from build123d import *

# Parameters (mm, degrees)
F0_R     = 4.953
F1_DEPTH = 4.7752
F2_DEPTH = 6.35
F4_DEPTH = 1.5748
F5_SIZE2 = 1.57479
F5_SIZE  = 3.17499
F6_SIZE  = 1.57479
F7_R     = 9.525
F8_R     = 4.953
F9_DEPTH = 6.35
F11_D    = 9.92124


# Not quite as in the source:
# - a fillet or chamfer is up to 0.001 mm smaller than in the source, because OpenCascade refuses the exact size


with BuildPart() as f1:
    # F0 (on Front) → F1 (new body)
    with BuildSketch(Plane.XZ):
        Polygon((0, 31.75), (0, 0), (25.4, 0), (25.4, 31.75), (12.7, 31.75), align=None)
        with BuildLine():
            ThreePointArc((22.225, 22.225), (5.9648079092, 15.4898079092), (12.7, 31.75))
            ThreePointArc((12.7, 31.75), (19.4351920908, 28.9601920908), (22.225, 22.225))
        make_face(mode=Mode.SUBTRACT)
        with BuildLine():
            ThreePointArc((22.225, 22.225), (19.4351920908, 28.9601920908), (12.7, 31.75))
            ThreePointArc((12.7, 31.75), (5.9648079092, 15.4898079092), (22.225, 22.225))
        make_face()
        with Locations((12.7, 22.225)):
            Circle(F0_R, mode=Mode.SUBTRACT)
    extrude(amount=F1_DEPTH)

    # F0 (on Front) → F2 (join)
    with BuildSketch(Plane.XZ):
        with BuildLine():
            ThreePointArc((22.225, 22.225), (19.4351920908, 28.9601920908), (12.7, 31.75))
            ThreePointArc((12.7, 31.75), (5.9648079092, 15.4898079092), (22.225, 22.225))
        make_face()
        with Locations((12.7, 22.225)):
            Circle(F0_R, mode=Mode.SUBTRACT)
    extrude(amount=F2_DEPTH)

    # F3 (on face) → F4 (join, through all)
    with BuildSketch(Plane.XZ.offset(6.35)):
        with BuildLine():
            ThreePointArc((25.4, 10.2581491177), (12.7, 4.7752), (0, 10.2581491177))
            Line((0, 10.2581491177), (0, 0))
            Line((0, 0), (25.4, 0))
            Line((25.4, 0), (25.4, 10.2581491177))
        make_face()
    extrude(amount=-F4_DEPTH)

    # F5 (size 3.175 and 1.5748 in the source; OpenCascade refuses exactly that, so slightly less here)
    f5_edges = [f1.edges().sort_by_distance(p)[0] for p in [
        (3.175, -6.35, 22.225),
    ]]
    f5_side = f1.faces().sort_by_distance((3.444408, -6.35, 22.225))[0]
    chamfer(f5_edges, length=F5_SIZE, length2=F5_SIZE2, reference=f5_side)

    # F6 (size 1.5748 in the source; OpenCascade refuses exactly that, so slightly less here)
    f6_edges = [f1.edges().sort_by_distance(p)[0] for p in [
        (12.7, -6.35, 4.7752),
    ]]
    chamfer(f6_edges, length=F6_SIZE)

    # F7
    f7_edges = [f1.edges().sort_by_distance(p)[0] for p in [
        (0, -2.3876, 31.75),
        (25.4, -2.3876, 31.75),
    ]]
    fillet(f7_edges, radius=F7_R)

    # F8 (on face) → F9 (join, through all)
    with BuildSketch(Plane.XZ.offset(6.35)):
        with Locations((12.7, 22.225)):
            Circle(F8_R)
    extrude(amount=-F9_DEPTH)

    # F11 (through all)
    with Locations(Plane.XZ.offset(6.35)):
        with Locations((12.7, 22.225)):
            Hole(F11_D / 2)


solid = f1.part
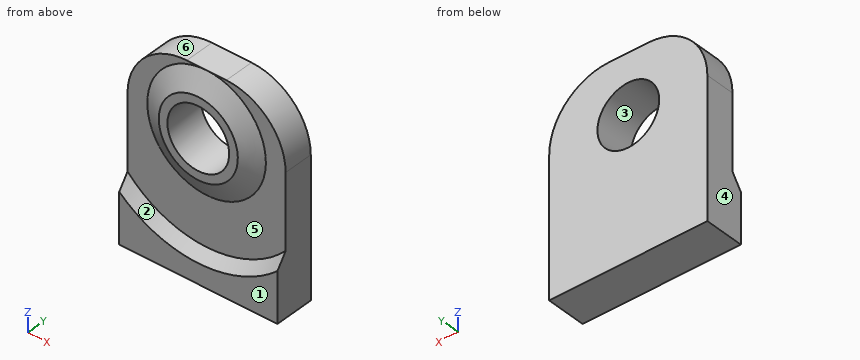
Input: part model. Units: mm. Frame: model coordinates. Face numbers are marked on the shaded views. A direction names the side the tool comes from. Give positions to 0.01 mm unless a question says otherwise; leave off trailing zeros. Write each loop counter-clockwise with the first axis right and the second up, starting at its lowest first coordinate (ties: lowest second). Pieces come first, ordered by that corner, then holes. Notation, with made-up numbers: M -12,64.25 L 44,64.25 A17 cw 44,89.25 Z; hole C 38,89.25 d3. An arc over 180 degrees is marked long. Write item = value, one per line. Start each with the question number.
1) Cut plane A-A on y = -3.75. Return the cut outline in (x, z) (3 decimals), then the cut area to 3 significant figures.
2) Draft query along X for the marked faces 1, 2, 3 and 4. Return one class per face: +X half, -X half, draft (parallel to the pull), parting line (faces both ways), or undercut.
3) Material intervals for line 1 along Z through (x, y) = (12.7, -3); line 2 along Y through (x, z) = (20, 11); line 3 along X through (y, z) = (-4.25, 24.5), sorted ascending. Write a range as [from, to].
4) First-contact query: pin 1 Ø7.5 at (x, z) = (17.5, 13) entering from -Y. Flat tip, straight axial feed; report the tip coordinate or a pass-through.
5) Reachability of the marked faces 5 and 6 from +Z, -Z, +X, -X, +Y, -Y: full face, straight path, thin tool, end or side. Return the list, or none.
Solved:
q1.outline = M 0,0 L 25.4,0 L 25.4,22.225 A9.525 ccw 15.875,31.75 L 9.525,31.75 A9.525 ccw 0,22.225 Z; hole C 12.7,22.225 d9.921
q1.area = 690 mm2
q2.face_1 = draft
q2.face_2 = undercut
q2.face_3 = undercut
q2.face_4 = -X half
q3.line_1 = [0, 17.26], [27.19, 31.75]
q3.line_2 = [-4.78, 0]
q3.line_3 = [0.28, 8.29], [17.11, 25.12]
q4.pin_1 = -6.2
q5.face_5 = -Y
q5.face_6 = +Z, -X, +Y, -Y
